```python
from build123d import *

# Parameters (mm, degrees)
BASE_EXTRUDE_DEPTH      = 20
FILLET1_R               = 10
CUT_EXTRUDE1_DEPTH      = 108.819293264
CUT_EXTRUDE1_DEPTH_BACK = 108.819293264
SKETCH2_R               = 7.5


with BuildPart() as part:
    # Sketch1 → Base-Extrude (new body)
    with BuildSketch(Plane.XY):
        Polygon((-80, 15), (-50, 15), (70, 35), (100, 35), (100, 20), (70, 20), (70, -10), (100, -10), (100, -25), (70, -25), (-50, -5), (-80, -5), align=None)
        Polygon((50, 21.528729116), (0, 13.195395783), (0, -3.195395783), (50, -11.528729116), align=None, mode=Mode.SUBTRACT)
    extrude(amount=BASE_EXTRUDE_DEPTH)

    # Fillet1
    # the kernel refuses this fillet: 10 mm, written as the material it takes off along each edge
    with BuildSketch(Plane(origin=(100, 60, 0), x_dir=(0, 0, 1), z_dir=(0, -1, 0)), Plane(origin=(100, 15, 0), x_dir=(0, 0, 1), z_dir=(0, -1, 0))) as fillet1_piece_1:
        with BuildLine():
            CenterArc((FILLET1_R, FILLET1_R), FILLET1_R, 180, 90)
            Line((0, FILLET1_R), (0, 0))
            Line((0, 0), (FILLET1_R, 0))
        make_face()
    extrude(amount=65, mode=Mode.SUBTRACT)
    with BuildSketch(Plane(origin=(-80, -30, 0), x_dir=(0, 0, 1), z_dir=(0, 1, 0))) as fillet1_piece_2:
        with BuildLine():
            CenterArc((FILLET1_R, FILLET1_R), FILLET1_R, 180, 90)
            Line((0, FILLET1_R), (0, 0))
            Line((0, 0), (FILLET1_R, 0))
        make_face()
    extrude(amount=70, mode=Mode.SUBTRACT)
    with BuildSketch(Plane(origin=(100, 15, 20), x_dir=(0, 0, -1), z_dir=(0, -1, 0)), Plane(origin=(100, 60, 20), x_dir=(0, 0, -1), z_dir=(0, -1, 0))) as fillet1_piece_3:
        with BuildLine():
            CenterArc((FILLET1_R, -FILLET1_R), FILLET1_R, 90, 90)
            Line((0, -FILLET1_R), (0, 0))
            Line((0, 0), (FILLET1_R, 0))
        make_face()
    extrude(amount=65, mode=Mode.SUBTRACT)
    with BuildSketch(Plane(origin=(-80, -30, 20), x_dir=(0, 0, -1), z_dir=(0, 1, 0))) as fillet1_piece_4:
        with BuildLine():
            CenterArc((FILLET1_R, -FILLET1_R), FILLET1_R, 90, 90)
            Line((0, -FILLET1_R), (0, 0))
            Line((0, 0), (FILLET1_R, 0))
        make_face()
    extrude(amount=70, mode=Mode.SUBTRACT)

    # Sketch2 → Cut-Extrude1 (cut, two sides: drawn at the far end of the back side and taken through both)
    with BuildSketch(Plane(origin=(0, 0, 0), x_dir=(1, 0, 0), z_dir=(0, 1, 0)).offset(-CUT_EXTRUDE1_DEPTH_BACK)):
        with Locations(Location((90, -10, 0), (0, 0, 270))):
            Circle(SKETCH2_R)
        with Locations(Location((-70, -10, 0), (0, 0, 270))):
            Circle(SKETCH2_R)
    extrude(amount=CUT_EXTRUDE1_DEPTH + CUT_EXTRUDE1_DEPTH_BACK, mode=Mode.SUBTRACT)


solid = part.part
```
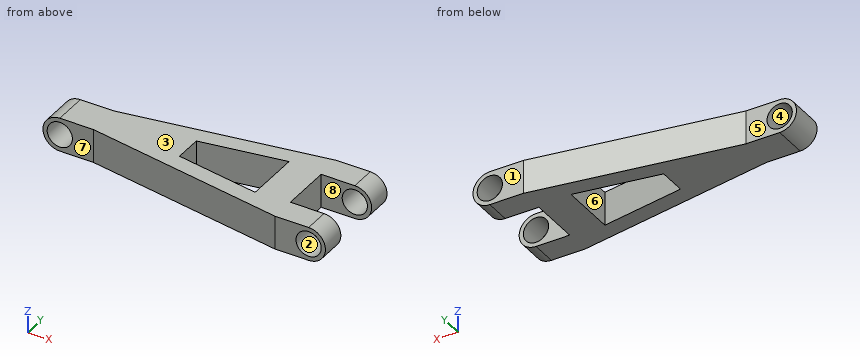
Build history of the part. All positions in model axes, mm. Face numbers are marked on the shaded views. A direction names the side the tool comes from. Round coordinates to 2 decimals unless told otherwise and drop trailing zeros. Loops run counter-clockwise (first coordinate to the right, second up) from the corner with the lowest first, then second, coordinate; pieces in that order, holes last.
Item 1: Drill centre lines: line 1 along X through (y, z) = (2.5, 10); line 2 along Z through (x, y) = (90, -16); line 3 along Y through (x, z) = (77, 17.5). Where is each one in solid material? Low to high.
Item 2: Two-plate mould, pull along Z, no slides. Class the marked faces 1, 2, 3 and 4: released by +Z, released by -Z, zero draft, split by the parting line, or undercut.
Item 3: Saw through at C-C (x = 86). List the corners of the cut face in (y, z), then the cut area to 3 significant figures.
Item 4: Saw through at A-A (y = 6). List the corners of the cut face in (x, z).
Item 5: Saw through at B-B (z = 10). List the corners of the cut face in (x, y), then the cut area to 3 significant figures.
Item 6: Saw through at D-D (x = 42.5). List the corners of the cut face in (y, z), then the cut area to 3 significant figures.
Item 7: Which spindle directions (+Z, -Z, +X, -X, +Y, -Y) get a long thin tool onto all of the face, cutting with end or side? Do the marked faces 5, 6, 7 and 8. Say none if no direction does.
Item 8: Pin check, flat tips, straight feed: P1, Ø3, axis at y = 28, z = 5.5, coming from the +X side; P2, Ø10, axis at x = -60, z = 15, coming from the +Y side; P3, Ø8, axis at y = 8, z = 14, coming from the +X side. Stop position of each tip, or through.
Worked answers:
1. line 1: x = -80 to -77.5, -62.5 to 0, 50 to 70
1. line 2: z = 0 to 2.5, 17.5 to 20
1. line 3: y = -25 to -10, 20 to 35
2. face 1: zero draft
2. face 2: undercut
2. face 3: released by +Z
2. face 4: undercut
3. outline: (-25, 0) - (-10, 0) - (-10, 3.66) - (-25, 3.66) - close; (-25, 16.34) - (-10, 16.34) - (-10, 20) - (-25, 20) - close; (20, 0) - (35, 0) - (35, 3.66) - (20, 3.66) - close; (20, 16.34) - (35, 16.34) - (35, 20) - (20, 20) - close
3. area: 219 mm2
4. outline: (-70, 0) - (0, 0) - (0, 20) - (-70, 20) arc R10 ccw to start; (50, 0) - (70, 0) - (70, 20) - (50, 20) - close; hole circle Ø15 at (-70, 10)
5. outline: (-80, -5) - (-77.5, -5) - (-77.5, 15) - (-80, 15) - close; (-62.5, -5) - (-50, -5) - (70, -25) - (82.5, -25) - (82.5, -10) - (70, -10) - (70, 20) - (82.5, 20) - (82.5, 35) - (70, 35) - (-50, 15) - (-62.5, 15) - close; (97.5, -25) - (100, -25) - (100, -10) - (97.5, -10) - close; (97.5, 20) - (100, 20) - (100, 35) - (97.5, 35) - close; hole (0, -3.2) - (50, -11.53) - (50, 21.53) - (0, 13.2) - close
5. area: 4,310 mm2
6. outline: (-20.42, 0) - (-10.28, 0) - (-10.28, 20) - (-20.42, 20) - close; (20.28, 0) - (30.42, 0) - (30.42, 20) - (20.28, 20) - close
6. area: 406 mm2
7. face 5: +Z, -Z, -X, +Y
7. face 6: +Z, -Z
7. face 7: +Z, -Z, -X, -Y
7. face 8: +Z, -Z, +X
8. P1: stops at x = 99.54
8. P2: stops at y = 15
8. P3: stops at x = 70
